Print and shaded views of the part. All mm, measured from the part's lowest x, y and z. A direction names the side the tool comes from. Coordinates: 2 decimals unless noted, no trailing zeros. Order: outer loops, then holes, each group sorted by start corner. A loop starts at its lowest first (then second) coordinate and runs counter-clockwise, first axis right, second up. Notation, with made-up numbers: M -2,43 L 14,43 A28 ccw 14,66 Z; hole C 76.25,9 d4. An arc over 180 degrees is marked long. One line per item, written item: value.
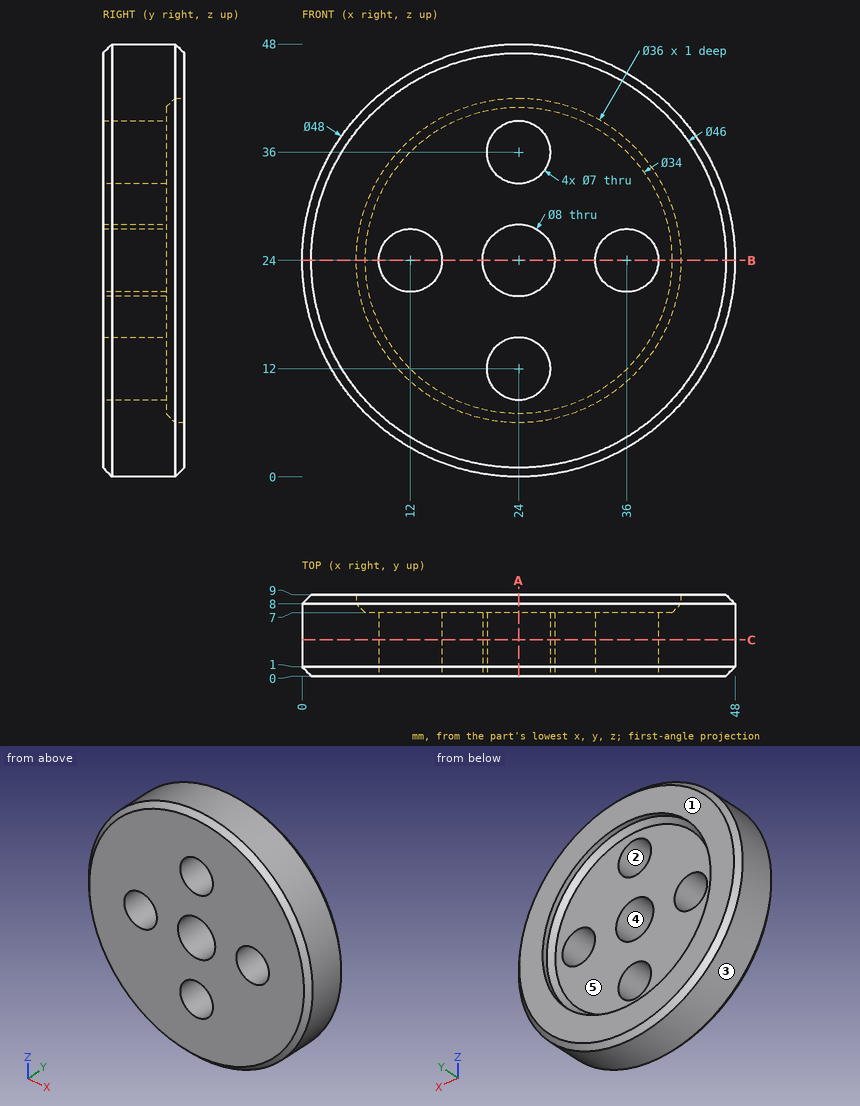
Q1. Mould opens along X. For the marked faces 1, 2 and 3 say: released by +X, released by -X, zero draft, split by the parting line, or undercut.
Recorded:
face 1: zero draft
face 2: undercut
face 3: split by the parting line
Q2. Drill centre lines: line 1 along X through (y, z) = (4.75, 24); line 2 along Y through (x, z) = (19, 9); line 3 along Z through (x, y) = (26, 2). Where is each one in solid material? Low to high.
Recorded:
line 1: x = 0 to 8.5, 15.5 to 20, 28 to 32.5, 39.5 to 48
line 2: y = 0 to 7
line 3: z = 0.08 to 9.13, 14.87 to 20.54, 27.46 to 33.13, 38.87 to 47.92
Q3. Slice it at C-C (y = 4). List the corners of the cut face in (x, z), plus the area to 3 significant figures.
Recorded:
outline: C 24,24 d48; hole C 12,24 d7; hole C 24,24 d8; hole C 24,12 d7; hole C 24,36 d7; hole C 36,24 d7
area: 1,610 mm^2
Q4. Pin check, flat tips, straight feed: pin 1 Ø1 at (x, z) = (15.5, 21) entering from +Y; pin 2 Ø6.5 at (x, z) = (24, 12) entering from +Y; pin 3 Ø5 at (y, z) = (1, 13) entering from +X; pin 4 Ø5 at (y, z) = (6.5, 20) entering from +X. Stop position of each tip, or through.
Recorded:
pin 1: stops at y = 7
pin 2: passes through
pin 3: stops at x = 46.44
pin 4: stops at x = 47.95
Q5. Slice it at B-B (z = 24). List the corners of the cut face in (x, y).
Recorded:
outline: M 0,1 L 1,0 L 8.5,0 L 8.5,7 L 7,7 L 6,8 L 6,9 L 1,9 L 0,8 Z; M 15.5,0 L 20,0 L 20,7 L 15.5,7 Z; M 28,0 L 32.5,0 L 32.5,7 L 28,7 Z; M 39.5,0 L 47,0 L 48,1 L 48,8 L 47,9 L 42,9 L 42,8 L 41,7 L 39.5,7 Z
Q6. Which spindle directions (+Z, -Z, +X, -X, +Y, -Y) get a long thin tool onto all of the face, cutting with end or side? Do the marked faces 4 and 5. Say none if no direction does.
Recorded:
face 4: +Y, -Y
face 5: +Y
Q7. Slice it at A-A (x = 24). List the corners of the cut face in (y, z).
Recorded:
outline: M 0,1 L 1,0 L 8,0 L 9,1 L 9,6 L 8,6 L 7,7 L 7,8.5 L 0,8.5 Z; M 0,15.5 L 7,15.5 L 7,20 L 0,20 Z; M 0,28 L 7,28 L 7,32.5 L 0,32.5 Z; M 0,39.5 L 7,39.5 L 7,41 L 8,42 L 9,42 L 9,47 L 8,48 L 1,48 L 0,47 Z
